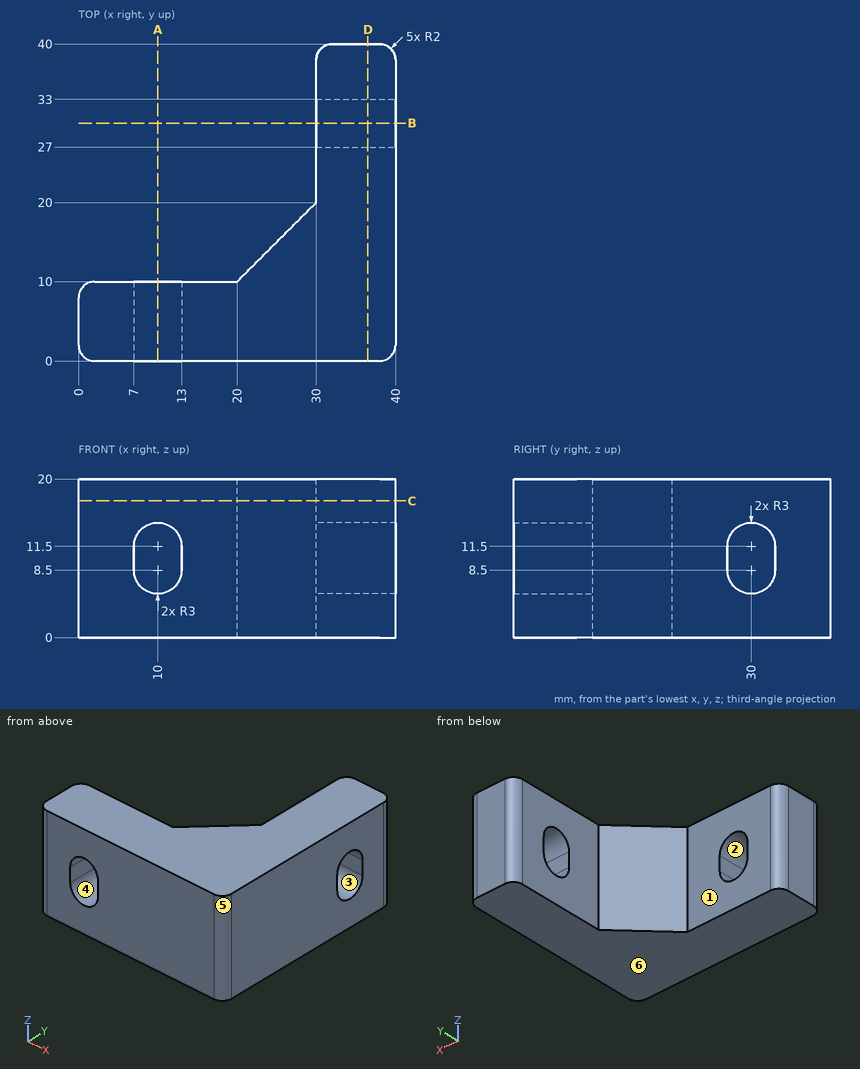
Source: three-view drawing plus pictorial views. Frame: mm from the lowest corner of the part. A direction names the side the tool comes from. Round coordinates to 2 decimals unless told otherwise and drop trailing zeros. Write each loop counter-clockwise with the first axis right and the second up, starting at its lowest first coordinate (ties: lowest second). Pieces come first, ordered by that corner, then holes. Notation, with made-up numbers: M 57.5,-32.75 L 63.5,-32.75 A33 cw 63.5,6.25 Z; hole C -38,-28.75 d7. An arc over 180 degrees is marked long. Write each question's results on one line, items separated by ' | '.
Q1. Section query B-B (y = 30). Return loops of the section in (x, z), and give its area (3 significant figures).
Results:
outline: M 30,0 L 40,0 L 40,5.5 L 30,5.5 Z; M 30,14.5 L 40,14.5 L 40,20 L 30,20 Z | area: 110 mm^2
Q2. Line query: line 1 along Y through (x, z) = (5.5, 1); line 2 along X through (y, z) = (3.5, 11.25); line 3 along X through (y, z) = (20.5, 11). Output: solid intervals per line, ascending.
Results:
line 1: y = 0 to 10 | line 2: x = 0 to 7, 13 to 40 | line 3: x = 30 to 40
Q3. Section query D-D (x = 36.5). Return loops of the section in (y, z), and give its area (3 significant figures).
Results:
outline: M 0,0 L 40,0 L 40,20 L 0,20 Z; hole M 27,8.5 A3 ccw 33,8.5 L 33,11.5 A3 ccw 27,11.5 Z | area: 754 mm^2
Q4. Pin query (flat end, axial travel): P1, Ø4, axis at x = 23, z = 4.5, coming from the +Y side. Return the tip coordinate at first contact, or that it passes through.
Results:
P1: stops at y = 15
Q5. Draft query along Z for the marked faces 4, 5 and 6. Return one class per face: released by +Z, released by -Z, zero draft, split by the parting line, or undercut.
Results:
face 4: undercut | face 5: zero draft | face 6: released by -Z
Q6. Section query A-A (x = 10). Return loops of the section in (y, z), and give its area (3 significant figures).
Results:
outline: M 0,0 L 10,0 L 10,5.5 L 0,5.5 Z; M 0,14.5 L 10,14.5 L 10,20 L 0,20 Z | area: 110 mm^2
Q7. Section query C-C (z = 17.25). Return loops of the section in (x, y), and give its area (3 significant figures).
Results:
outline: M 0,2 A2 ccw 2,0 L 38,0 A2 ccw 40,2 L 40,38 A2 ccw 38,40 L 32,40 A2 ccw 30,38 L 30,20 L 20,10 L 2,10 A2 ccw 0,8 Z | area: 746 mm^2
Q8. Access query for the marked faces 1, 2 and 3. Directions: +Z, -Z, +X, -X, +Y, -Y. A direction counts if a zero-diameter tool reaches every point of the face in a straight line with its end or side. Return the directions, or none.
Results:
face 1: +Z, -Z, -X, +Y | face 2: +Y, -Y | face 3: +X, -X
